Verification items for the finished model (mm, model axes). A direction names the side the tool comes from. Coordinates: 2 decimals unless noted, no trailing zeros. Order: outer loops, then holes, each group sorted by start corner. A loop starts at its lowest first (then second) coordinate and runs counter-clockwise, first axis right, second up. Notation, with made-up numbers: (29.5, 67.25) -> (86.5, 67.25) arc R8 cw to (86.5, 74.25) -> close; hole circle Ø2 at (-5.75, 22.5). An arc over 180 degrees is marked (long way). Write each question's results on one line, items separated by ' | '. Start each with the question number.
(1) Cross-section at C-C on z = 100. Enter the section's corners in (x, y), and give its area (3 significant figures).
(2) Draft check along X on faces 3 (the flat face through (77.5, -3, 158)), 4 (the flat face through (50, -46, 74)), 5 (the flat face through (-77.5, -3, 158)), 6 (the flat face through (-1, 3, 320.16)). Enter one of: +X half, -X half, draft (parallel to the pull), parting line (faces both ways), or undercut.
(3) Set-up check for faces 1 (the flat face through (-1, 195, 158)), 2 (the flat face through (-50, -46, 74)): record each of +Z, -Z, +X, -X, +Y, -Y from which the full face is reachable in a straight line by a thin tool's end or side.
(4) Cross-section at B-B on y = -45. Enter the section's corners in (x, z), and give its area (3 significant figures).
(5) Thickness scan on probe 1 along X at (y, z) = (-23.5, 92.5); probe 2 along Y at (x, z) = (-8.5, 37); probe 3 along Z at (x, y) = (-69, -45). Record the ranges inside material, lowest first. Write a range as [from, to].
(6) Cross-section at D-D on x = 43.5. Enter the section's corners in (y, z), and give its area (3 significant figures).
(7) Cross-section at A-A on z = 45.5. Enter the section's corners in (x, y), and give its area (4 significant figures).
```python
from build123d import *

# Parameters (mm, degrees)
SKETCH1_W               = 155
SKETCH1_H               = 390
BOSS_EXTRUDE1_DEPTH     = 320.16
SKETCH2_W               = 100
SKETCH2_H               = 100
CUT_EXTRUDE1_DEPTH      = 150
CUT_EXTRUDE2_DEPTH      = 406.650620115
CUT_EXTRUDE2_DEPTH_BACK = 406.650620115
SKETCH3_R               = 15


with BuildPart() as part:
    # Sketch1 → Boss-Extrude1 (new body)
    with BuildSketch(Plane.XY):
        Rectangle(SKETCH1_W, SKETCH1_H)
    extrude(amount=BOSS_EXTRUDE1_DEPTH)

    # Sketch2 → Cut-Extrude1 (cut)
    with BuildSketch(Plane(origin=(0, 0, 0), x_dir=(-1, 0, 0), z_dir=(0, 0, -1))):
        with Locations((0, -45)):
            Rectangle(SKETCH2_W, SKETCH2_H)
    extrude(amount=-CUT_EXTRUDE1_DEPTH, mode=Mode.SUBTRACT)

    # Sketch3 → Cut-Extrude2 (cut, two sides: drawn at the far end of the back side and taken through both)
    with BuildSketch(Plane(origin=(77.5, 0, 0), x_dir=(0, 0, -1), z_dir=(1, 0, 0)).offset(-CUT_EXTRUDE2_DEPTH_BACK)):
        with Locations(Location((-100, -45, 0), (0, 0, 90))):
            Circle(SKETCH3_R)
    extrude(amount=CUT_EXTRUDE2_DEPTH + CUT_EXTRUDE2_DEPTH_BACK, mode=Mode.SUBTRACT)


solid = part.part
```
Results are:
1) outline: (-77.5, -195) -> (77.5, -195) -> (77.5, -60) -> (50, -60) -> (50, -95) -> (-50, -95) -> (-50, -60) -> (-77.5, -60) -> close; (-77.5, -30) -> (-50, -30) -> (-50, 5) -> (50, 5) -> (50, -30) -> (77.5, -30) -> (77.5, 195) -> (-77.5, 195) -> close | area: 48,800 mm2
2) face 3: +X half | face 4: undercut | face 5: -X half | face 6: draft
3) face 1: +Z, -Z, +X, -X, +Y | face 2: -Z
4) outline: (-77.5, 0) -> (-50, 0) -> (-50, 85) -> (-77.5, 85) -> close; (-77.5, 115) -> (-50, 115) -> (-50, 150) -> (50, 150) -> (50, 115) -> (77.5, 115) -> (77.5, 320.16) -> (-77.5, 320.16) -> close; (50, 0) -> (77.5, 0) -> (77.5, 85) -> (50, 85) -> close | area: 33,000 mm2
5) probe 1: x = [-77.5, -50], [50, 77.5] | probe 2: y = [-195, -95], [5, 195] | probe 3: z = [0, 85], [115, 320.16]
6) outline: (-195, 0) -> (-95, 0) -> (-95, 150) -> (5, 150) -> (5, 0) -> (195, 0) -> (195, 320.16) -> (-195, 320.16) -> close | area: 110,000 mm2
7) outline: (-77.5, -195) -> (77.5, -195) -> (77.5, 195) -> (-77.5, 195) -> close; hole (-50, -95) -> (50, -95) -> (50, 5) -> (-50, 5) -> close | area: 50,450 mm2
